For this review, take the finished solid that the model builds, in its own axes (mm). Face numbers are marked on the shaded views. A direction names the side the tool comes from. Coordinates: 2 decimals unless noted, no trailing zeros. One line per item, written item: value. Start each with the question number.
(1) To check wall thickness, follow line 1 along Y through (x, z) = (0, 45.05); line 2 along X through (y, z) = (25.4, 46.95); line 3 along Y through (x, z) = (1.5, 45.5). State the ranges of each line that lie inside material, in increasing order.
(2) Clearance check with flat-ended pins moving along their axes: pin 1 (3 mm diameter, centred on x = -1.5, z = 47, fed in from -Y); pin 2 (1.5 mm diameter, centred on x = 2, z = 28.5, fed in from -Y); pin 3 (2 mm diameter, centred on x = -3.5, z = 32.5, fed in from +Y); pin 4 (4.5 mm diameter, centred on x = 0.5, y = 0, fed in from -Z). State where each tip first meets the part, or that it passes through.
(3) Consider section A-A on y = -25.4. Count the separate pieces of the cut face and the enclosed holes in it, then the cut area to 3 significant figures.
(4) Mouldability with a two-part tool opening along Y and no side actions: class the marked faces 1 and 2 as released by +Y, released by -Y, zero draft, split by the parting line, or undercut.
(5) For the marked faces 3 and 4, list the 3-axis set-ups (+Z, -Z, +X, -X, +Y, -Y) from which the entire face can be reached by the end or side of a thin tool; tool diameter is ignored.
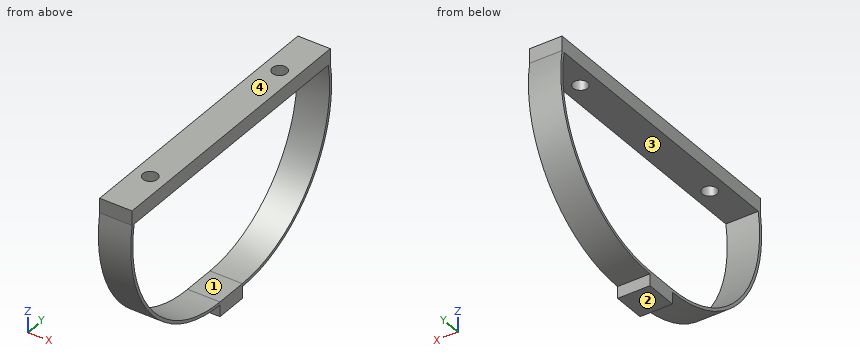
Autodesk Inventor part; units mm, degrees
ref_plane "YZ Plane" through (0, 0, 0) normal (1, 0, 0) x (0, 1, 0)
ref_plane "XZ Plane" through (0, 0, 0) normal (0, 1, 0) x (-1, 0, 0)
ref_plane "XY Plane" through (0, 0, 0) normal (0, 0, 1) x (1, 0, 0)
sketch "Sketch1" plane through (0, 0, 0) normal (0, 0, 1) x (1, 0, 0)
  circle A0 centre (0, 0) radius 2
  arc A1 (3.5334, 2.622) -> (3.5334, -2.622) centre (0, 0) ccw
  spline S0 degree 3 poles (3.5334, -2.622) (3.7278, -2.3601) (3.9365, -2.0888) (4.2711, -1.5149) (4.4221, -1.1997) (4.5595, -0.6718) (4.5884, -0.5166) (4.6147, -0.2815) (4.6206, -0.2033) (4.626, -0.0622) (4.6266, 0.0005) (4.624, 0.1338) (4.6203, 0.2042) (4.6043, 0.3928) (4.5877, 0.5103) (4.479, 1.0643) (4.3163, 1.4256) (3.965, 2.0517) (3.7411, 2.3422) (3.5334, 2.622) knots 0 0 0 0 0.091406 0.091406 0.164876 0.164876 0.194861 0.194861 0.209742 0.209742 0.221646 0.221646 0.235028 0.235028 0.25755 0.25755 0.34212 0.34212 0.446672 0.446672 0.446672 0.446672
  line L0 (4.4, -4.4) -> (-4.4, -4.4)
  line L1 (-4.4, -4.4) -> (-4.4, 4.4)
  line L2 (-4.4, 4.4) -> (4.4, 4.4)
  line L3 (4.4, 4.4) -> (4.4, -4.4)
  line L4 (4.4, -4.4) -> (-4.4, 4.4) construction
  line L5 (-4.4, -4.4) -> (4.4, 4.4) construction
  point P0 (0, 0)
extrude "Extrusion1" add sketch "Sketch1" along normal blind 4 contours A0 | S0 L3 A1 | A1 L2 L3 S0 | A1 L1 L2 | A1 L0 L1 | L3 L0 A1 S0
ref_plane "Work Plane1" through (-30.8084, 0, 48.1765) normal (0, 0, 1) x (1, 0, 0)
sketch "Sketch2" plane through (-30.8084, 0, 48.1765) normal (0, 0, 1) x (1, 0, 0)
  line L0 (35.2084, 38.1) -> (26.4084, 38.1)
  line L1 (26.4084, 38.1) -> (26.4084, -38.1)
  line L2 (26.4084, -38.1) -> (35.2084, -38.1)
  line L3 (35.2084, -38.1) -> (35.2084, 38.1)
  line L4 (35.2084, 38.1) -> (26.4084, -38.1) construction
  line L5 (26.4084, 38.1) -> (35.2084, -38.1) construction
  line L6 (35.2084, 4.4) -> (26.4084, 4.4)
  line L7 (26.4084, 4.4) -> (26.4084, -4.4)
  line L8 (26.4084, -4.4) -> (35.2084, -4.4)
  line L9 (35.2084, -4.4) -> (35.2084, 4.4)
  line L10 (35.2084, -38.1) -> (26.4084, -38.1)
  line L11 (26.4084, -38.1) -> (26.4084, -38.9)
  line L12 (26.4084, -38.9) -> (35.2084, -38.9)
  line L13 (35.2084, -38.9) -> (35.2084, -38.1)
  line L14 (35.2084, 38.1) -> (26.4084, 38.1)
  line L15 (26.4084, 38.1) -> (26.4084, 38.9)
  line L16 (26.4084, 38.9) -> (35.2084, 38.9)
  line L17 (35.2084, 38.9) -> (35.2084, 38.1)
  point P0 (30.8084, 0)
  point P1 (26.4084, 0)
  point P2 (26.4084, -38.1)
  dimension "d2" = 38.1
  dimension "d8" = 0.8
  dimension "d9" = 0.8
sketch "Sketch4" plane through (-4.4, 4.4, 0) normal (0, 1, 0) x (1, 0, 0)
  line L0 (8.8, 0) -> (8.8, -4)
  line L1 (0, 0) -> (0, -4)
  line L2 (8.8, -4) -> (0, -4)
  line L3 (0, -4) -> (0, -3.2)
  line L4 (0, -3.2) -> (8.8, -3.2)
  line L5 (8.8, -3.2) -> (8.8, -4)
  point P0 (4.4, 0)
  dimension "d3" = 0.8
extrude "Extrusion2" add sketch "Sketch2" against normal blind 4
sketch "Sketch3" plane through (4.4, -4.4, 0) normal (1, 0, 0) x (0, 0, -1)
  line L0 (-48.1765, -33.7) -> (-48.1765, 42.5) construction
  line L1 (0, 0) -> (0, 8.8)
  line L2 (0, 8.8) -> (-4, 8.8)
  line L3 (-4, 0) -> (-4, 8.8)
  line L4 (0, 0) -> (-4, 0)
  arc A0 (-44.1765, -33.7) -> (-4, 0) centre (-38.222, 0) ccw
  line L5 (-44.1765, 43.3) -> (-44.1765, -34.5)
  arc A1 (-4, 8.8) -> (-44.1765, 42.5) centre (-38.222, 8.8) ccw
  line L6 (-44.1765, -33.7) -> (-44.1765, 42.5)
  point P0 (0, 4.4)
sweep "Sweep2" add profiles "Sketch4" path "Sketch3" path curves A1 L6 A0
sketch "Sketch5" plane through (-30.8084, 0, 48.1765) normal (0, 0, 1) x (1, 0, 0)
  line L0 (35.2084, -38.9) -> (35.2084, 38.9)
  line L1 (35.2084, 38.9) -> (26.4084, 38.9)
  line L2 (26.4084, 38.9) -> (26.4084, -38.9)
  line L3 (26.4084, -38.9) -> (35.2084, -38.9)
  circle A0 centre (30.8084, -25.4) radius 2
  line L4 (35.2084, 0) -> (26.4084, 0)
  circle A1 centre (30.8084, 25.4) radius 2
  point P0 (30.8084, 0)
  dimension "d12" = 4
  dimension "d13" = 25.4
hole "Hole1" at (0, -25.4, 48.1765) at (0, 25.4, 48.1765) direction (0, 0, -1) diameter 4 depth 6
properties part number "MotorMountBackSuspension"
Geometry check:
1. line 1: y = -38.9 to -27.4, -23.4 to 23.4, 27.4 to 38.9
1. line 2: x = -4.4 to -2, 2 to 4.4
1. line 3: y = -38.9 to -26.72, -24.08 to 24.08, 26.72 to 38.9
2. pin 1: stops at y = -38.9
2. pin 2: stops at y = -38.25
2. pin 3: stops at y = 39.1
2. pin 4: stops at z = 0
3. separate pieces: 3
3. enclosed holes: 0
3. area: 28.1 mm^2
4. face 1: undercut
4. face 2: zero draft
5. face 3: +X, -X
5. face 4: +Z, +X, -X, +Y, -Y
